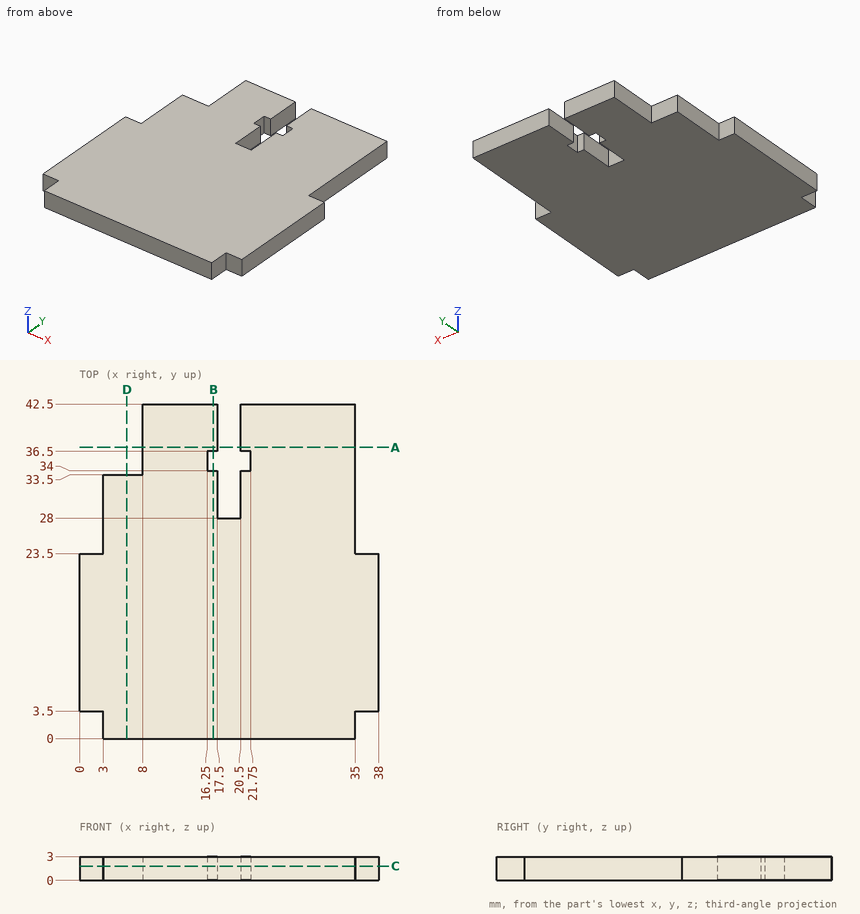
For this review, use the dimensioned drawing (mm, ordinates from the lowest corner) and the shaded views. Coordinates: 2 decimals unless noted, no trailing zeros. Order: outer loops, then holes, each group sorted by start corner. A loop starts at its lowest first (then second) coordinate and runs counter-clockwise, first axis right, second up. Notation, with made-up numbers: M -4.5,27 L 4.5,27 A13 cw 4.5,49 Z; hole C 40,83.25 d11. An arc over 180 degrees is marked long. Answer as a JSON object with one key per item and string values. Group by question number.
1) Add section A-A, the plane y = 37. Write out the cut boundary in (x, z).
2) Add section B-B, the plane x = 17. Write out the cut boundary in (y, z), then the cut area to 3 significant figures.
3) Add section C-C, the plane z = 1.8. Write out the cut boundary in (x, y), then the cut area to 3 significant figures.
4) For pin 1 (1.5 mm diameter, centred on y = 1.5, z = 1.5, fed in from +X); pin 2 (0.9 mm diameter, centred on x = 1, z = 1.5, fed in from -Y); pin 3 (1.5 mm diameter, centred on x = 19.5, z = 1.5, fed in from +Y), all flat-tipped, find the tip position at first contact; note any pin that passes through.
5) Wall thickness on L1, parallel to Y at x = 17, z = 0.9; L2, parallel to X at y = 30.5, z = 0.6; L3, parallel to X at y = 35, z = 0.85: over which ranges is each line inside the solid? List them lowest first.
6) Add section D-D, the plane x = 6. Write out the cut boundary in (y, z).
Computed values:
{
 "1": {"outline": "M 8,0 L 17.5,0 L 17.5,3 L 8,3 Z; M 20.5,0 L 35,0 L 35,3 L 20.5,3 Z"},
 "2": {"outline": "M 0,0 L 34,0 L 34,3 L 0,3 Z; M 36.5,0 L 42.5,0 L 42.5,3 L 36.5,3 Z", "area": "120 mm^2"},
 "3": {"outline": "M 0,3.5 L 3,3.5 L 3,0 L 35,0 L 35,3.5 L 38,3.5 L 38,23.5 L 35,23.5 L 35,42.5 L 20.5,42.5 L 20.5,36.5 L 21.75,36.5 L 21.75,34 L 20.5,34 L 20.5,28 L 17.5,28 L 17.5,34 L 16.25,34 L 16.25,36.5 L 17.5,36.5 L 17.5,42.5 L 8,42.5 L 8,33.5 L 3,33.5 L 3,23.5 L 0,23.5 Z", "area": "1,390 mm^2"},
 "4": {"pin 1": "stops at x = 35", "pin 2": "stops at y = 3.5", "pin 3": "stops at y = 28"},
 "5": {"L1": "y = 0 to 34, 36.5 to 42.5", "L2": "x = 3 to 17.5, 20.5 to 35", "L3": "x = 8 to 16.25, 21.75 to 35"},
 "6": {"outline": "M 0,0 L 33.5,0 L 33.5,3 L 0,3 Z"}
}
